CAD build for the part. Positions are in the model's coordinates, mm. A direction names the side the tool comes from. Round coordinates to 2 decimals unless told otherwise and drop trailing zeros. Loops run counter-clockwise (first coordinate to the right, second up) from the corner with the lowest first, then second, coordinate; pieces in that order, holes last. Notation, with made-up numbers: M 67,8 L 91,8 A35 ccw 91,40 Z; hole C 85.25,10.25 d7. An arc over 180 degrees is marked long. Use a Markdown table: item, result. Add a question column.
(1) Flat gauge pins, fed straight in: P1, Ø19.5, axis at x = -40, y = 0, coming from the +Z side; P2, Ø24, axis at y = 0, z = 124.5, coming from the -X side; P3, Ø10, axis at x = 27, y = -36, coming from the -Z side. Where does each tip first touch, or does it go through?
(2) Band-saw the part on C-C, the plane x = 0. Write the cut outline in (y, z), and give its area (3 significant figures).
(3) Band-saw the part on D-D, the plane z = 87. Write the cut outline in (x, y).
(4) Band-saw the part on B-B, the plane z = 117. Write the cut outline in (x, y).
(5) Which spindle directions (+Z, -Z, +X, -X, +Y, -Y) get a long thin tool onto all of the face, cutting with end or side? Do faces 3 (the face through (70, -1, -4)), 4 (the face through (-70, -1, 66)), 5 (the face through (20, -3.05, 2)). Say none if no direction does.
(6) Wall check: L1, parallel to Y at x = 0, z = 1.45; L2, parallel to Z at x = 72, y = 0; L3, parallel to X at y = 0, z = 1. Give the ranges that are in metal, low to high.
(7) Band-saw the part on A-A, the plane x = -40. Write the cut outline in (y, z), and give its area (3 significant figures).
(8) Two-plate mould, pull along X, no slides. Class faces 1 (the face through (72.218, 56.403, 77.65)), 2 (the face through (27.95, 0.07, 2.22)): released by +X, released by -X, zero draft, split by the parting line, or undercut.
from build123d import *

# Parameters (mm, degrees)
F0_W     = 140
F0_H     = 160
F0_R     = 6.05
F1_DEPTH = 4.5
F2_R     = 4
F2_R_2   = 10.35
F3_DEPTH = 4.5


with BuildPart() as f1:
    # F0 (on Top) → F1 (new body)
    with BuildSketch(Plane.XY):
        Rectangle(F0_W, F0_H)
        with Locations((0, -40)):
            Circle(F0_R, mode=Mode.SUBTRACT)
        with BuildLine():
            ThreePointArc((3.05, -24.9), (0, -27.95), (-3.05, -24.9))
            Line((-3.05, -24.9), (-3.05, -15.1))
            ThreePointArc((-3.05, -15.1), (0, -12.05), (3.05, -15.1))
            Line((3.05, -15.1), (3.05, -24.9))
        make_face(mode=Mode.SUBTRACT)
        with Locations((-40, 0)):
            Circle(F0_R, mode=Mode.SUBTRACT)
        with BuildLine():
            ThreePointArc((-24.9, -3.05), (-27.95, 0), (-24.9, 3.05))
            Line((-24.9, 3.05), (-15.1, 3.05))
            ThreePointArc((-15.1, 3.05), (-12.05, 0), (-15.1, -3.05))
            Line((-15.1, -3.05), (-24.9, -3.05))
        make_face(mode=Mode.SUBTRACT)
        Circle(F0_R, mode=Mode.SUBTRACT)
        with BuildLine():
            ThreePointArc((24.9, 3.05), (27.95, 0), (24.9, -3.05))
            Line((24.9, -3.05), (15.1, -3.05))
            ThreePointArc((15.1, -3.05), (12.05, 0), (15.1, 3.05))
            Line((15.1, 3.05), (24.9, 3.05))
        make_face(mode=Mode.SUBTRACT)
        with BuildLine():
            ThreePointArc((-3.05, 24.9), (0, 27.95), (3.05, 24.9))
            Line((3.05, 24.9), (3.05, 15.1))
            ThreePointArc((3.05, 15.1), (0, 12.05), (-3.05, 15.1))
            Line((-3.05, 15.1), (-3.05, 24.9))
        make_face(mode=Mode.SUBTRACT)
        with Locations((40, 0)):
            Circle(F0_R, mode=Mode.SUBTRACT)
        with Locations((0, 40)):
            Circle(F0_R, mode=Mode.SUBTRACT)
    extrude(amount=F1_DEPTH)

    # F2 (on face) → F3 (join)
    with BuildSketch(Plane.YZ.offset(70)):
        with BuildLine():
            Line((22.7183887259, 159.5), (-22.7183887259, 159.5))
            ThreePointArc((-22.7183887259, 159.5), (-28.6048019805, 157.5839432826), (-32.2354749035, 152.5700277992))
            Line((-32.2354749035, 152.5700277992), (-79.9034172355, 4.7994065699))
            ThreePointArc((-79.9034172355, 4.7994065699), (-79.9757067686, 4.496178687), (-80, 4.18540101))
            Line((-80, 4.18540101), (-80, -6.5))
            ThreePointArc((-80, -6.5), (-79.4142135624, -7.9142135624), (-78, -8.5))
            Line((-78, -8.5), (78, -8.5))
            ThreePointArc((78, -8.5), (79.4142135624, -7.9142135624), (80, -6.5))
            Line((80, -6.5), (80, 4.18540101))
            ThreePointArc((80, 4.18540101), (79.9757067686, 4.496178687), (79.9034172355, 4.7994065699))
            Line((79.9034172355, 4.7994065699), (32.2354749035, 152.5700277992))
            ThreePointArc((32.2354749035, 152.5700277992), (28.6048019805, 157.5839432826), (22.7183887259, 159.5))
        make_face()
        with Locations((0, 104.5)):
            Circle(F2_R, mode=Mode.SUBTRACT)
        with Locations((0, 124.5)):
            Circle(F2_R_2, mode=Mode.SUBTRACT)
        with Locations((0, 150.5)):
            Circle(F2_R, mode=Mode.SUBTRACT)
    extrude(amount=F3_DEPTH)

    # F4: F1 across plane


with BuildPart() as f1_1:
    add(f1.part)
    add(f1.part.mirror(Plane.YZ))


solid = f1_1.part
Return value:
| question | item | result |
|---|---|---|
| 1 | P1 | z = 4.5 |
| 1 | P2 | x = -74.5 |
| 1 | P3 | z = 0 |
| 2 | outline | M -80,0 L -46.05,0 L -46.05,4.5 L -80,4.5 Z; M -33.95,0 L -27.95,0 L -27.95,4.5 L -33.95,4.5 Z; M -12.05,0 L -6.05,0 L -6.05,4.5 L -12.05,4.5 Z; M 6.05,0 L 12.05,0 L 12.05,4.5 L 6.05,4.5 Z; M 27.95,0 L 33.95,0 L 33.95,4.5 L 27.95,4.5 Z; M 46.05,0 L 80,0 L 80,4.5 L 46.05,4.5 Z |
| 2 | area | 414 mm^2 |
| 3 | outline | M -74.5,-53.39 L -70,-53.39 L -70,53.39 L -74.5,53.39 Z; M 70,-53.39 L 74.5,-53.39 L 74.5,53.39 L 70,53.39 Z |
| 4 | outline | M -74.5,-43.71 L -70,-43.71 L -70,-7.13 L -74.5,-7.13 Z; M -74.5,7.13 L -70,7.13 L -70,43.71 L -74.5,43.71 Z; M 70,-43.71 L 74.5,-43.71 L 74.5,-7.13 L 70,-7.13 Z; M 70,7.13 L 74.5,7.13 L 74.5,43.71 L 70,43.71 Z |
| 5 | face 3 | -Z, +Y, -Y |
| 5 | face 4 | +Z, +Y, -Y |
| 5 | face 5 | +Z, -Z |
| 6 | L1 | -80 to -46.05, -33.95 to -27.95, -12.05 to -6.05, 6.05 to 12.05, 27.95 to 33.95, 46.05 to 80 |
| 6 | L2 | -8.5 to 100.5, 108.5 to 114.15, 134.85 to 146.5, 154.5 to 159.5 |
| 6 | L3 | -74.5 to -46.05, -33.95 to -27.95, -12.05 to -6.05, 6.05 to 12.05, 27.95 to 33.95, 46.05 to 74.5 |
| 7 | outline | M -80,0 L -6.05,0 L -6.05,4.5 L -80,4.5 Z; M 6.05,0 L 80,0 L 80,4.5 L 6.05,4.5 Z |
| 7 | area | 666 mm^2 |
| 8 | face 1 | zero draft |
| 8 | face 2 | undercut |
